from build123d import *

# Parameters (mm, degrees)
SKETCH1_W                                      = 50.8
SKETCH1_H                                      = 50.8
BOSS_EXTRUDE1_DEPTH                            = 6.35
CUT_EXTRUDE1_REACH                             = 38.478
SKETCH2_R                                      = 4.7625
SKETCH2_R_2                                    = 3.175
CUT_EXTRUDE2_REACH                             = 38.478
SKETCH5_R                                      = 1.4732
CSK_FOR_4_FLAT_HEAD_MACHINE_SCREW1_D           = 2.9464
CSK_FOR_4_FLAT_HEAD_MACHINE_SCREW1_CSINK_D     = 5.715
CSK_FOR_4_FLAT_HEAD_MACHINE_SCREW1_CSINK_ANGLE = 82
FILLET1_R                                      = 0.635


with BuildPart() as part:
    # Sketch1 → Boss-Extrude1 (new body)
    with BuildSketch(Plane(origin=(0, 0, 0), x_dir=(0, 1, 0), z_dir=(0, 0, 1))):
        Rectangle(SKETCH1_W, SKETCH1_H)
    extrude(amount=BOSS_EXTRUDE1_DEPTH)

    # Sketch2 → Cut-Extrude1 (cut, up to next)
    with BuildSketch(Plane.XY.offset(6.35), mode=Mode.PRIVATE) as cut_extrude1_sk1:
        with Locations((0, 8.73125)):
            Circle(SKETCH2_R)
    cut_extrude1_tool1 = extrude(cut_extrude1_sk1.sketch, amount=-CUT_EXTRUDE1_REACH, mode=Mode.PRIVATE) & part.part
    # Sketch2 → Cut-Extrude1 (cut, up to next)
    with BuildSketch(Plane.XY.offset(6.35), mode=Mode.PRIVATE) as cut_extrude1_sk2:
        with Locations((0, -8.73125)):
            Circle(SKETCH2_R_2)
    cut_extrude1_tool2 = extrude(cut_extrude1_sk2.sketch, amount=-CUT_EXTRUDE1_REACH, mode=Mode.PRIVATE) & part.part
    add(cut_extrude1_tool1.solids().sort_by_distance((0, 8.73125, 6.35))[0], mode=Mode.SUBTRACT)
    add(cut_extrude1_tool2.solids().sort_by_distance((0, -8.73125, 6.35))[0], mode=Mode.SUBTRACT)

    # Sketch5 → Cut-Extrude2 (cut, up to next)
    with BuildSketch(Plane.XY.offset(6.35), mode=Mode.PRIVATE) as cut_extrude2_sk1:
        with Locations((-20.32, 20.32)):
            Circle(SKETCH5_R)
    cut_extrude2_tool1 = extrude(cut_extrude2_sk1.sketch, amount=-CUT_EXTRUDE2_REACH, mode=Mode.PRIVATE) & part.part
    # Sketch5 → Cut-Extrude2 (cut, up to next)
    with BuildSketch(Plane.XY.offset(6.35), mode=Mode.PRIVATE) as cut_extrude2_sk2:
        with Locations((20.32, 20.32)):
            Circle(SKETCH5_R)
    cut_extrude2_tool2 = extrude(cut_extrude2_sk2.sketch, amount=-CUT_EXTRUDE2_REACH, mode=Mode.PRIVATE) & part.part
    # Sketch5 → Cut-Extrude2 (cut, up to next)
    with BuildSketch(Plane.XY.offset(6.35), mode=Mode.PRIVATE) as cut_extrude2_sk3:
        with Locations((-20.32, -20.32)):
            Circle(SKETCH5_R)
    cut_extrude2_tool3 = extrude(cut_extrude2_sk3.sketch, amount=-CUT_EXTRUDE2_REACH, mode=Mode.PRIVATE) & part.part
    # Sketch5 → Cut-Extrude2 (cut, up to next)
    with BuildSketch(Plane.XY.offset(6.35), mode=Mode.PRIVATE) as cut_extrude2_sk4:
        with Locations((20.32, -20.32)):
            Circle(SKETCH5_R)
    cut_extrude2_tool4 = extrude(cut_extrude2_sk4.sketch, amount=-CUT_EXTRUDE2_REACH, mode=Mode.PRIVATE) & part.part
    add(cut_extrude2_tool1.solids().sort_by_distance((-20.32, 20.32, 6.35))[0], mode=Mode.SUBTRACT)
    add(cut_extrude2_tool2.solids().sort_by_distance((20.32, 20.32, 6.35))[0], mode=Mode.SUBTRACT)
    add(cut_extrude2_tool3.solids().sort_by_distance((-20.32, -20.32, 6.35))[0], mode=Mode.SUBTRACT)
    add(cut_extrude2_tool4.solids().sort_by_distance((20.32, -20.32, 6.35))[0], mode=Mode.SUBTRACT)

    # CSK for #4 Flat Head Machine Screw1 (through all)
    with Locations(Plane.XY.offset(6.35)):
        with Locations((-20.32, 20.32), (20.32, 20.32), (20.32, -20.32), (-20.32, -20.32)):
            CounterSinkHole(CSK_FOR_4_FLAT_HEAD_MACHINE_SCREW1_D / 2, CSK_FOR_4_FLAT_HEAD_MACHINE_SCREW1_CSINK_D / 2, counter_sink_angle=CSK_FOR_4_FLAT_HEAD_MACHINE_SCREW1_CSINK_ANGLE)

    # Fillet1
    fillet1_edges = [part.edges().sort_by_distance(p)[0] for p in [
        (0, -25.4, 6.35),
        (25.4, 0, 6.35),
        (0, 25.4, 6.35),
        (25.4, 0, 0),
        (0, -25.4, 0),
        (-25.4, 0, 0),
        (0, 25.4, 0),
        (25.4, 25.4, 3.175),
        (25.4, -25.4, 3.175),
        (-25.4, -25.4, 3.175),
        (-25.4, 25.4, 3.175),
        (-25.4, 0, 6.35),
    ]]
    fillet(fillet1_edges, radius=FILLET1_R)


solid = part.part
Part model, mm, in its own coordinate system. Coordinates: 2 decimals unless noted, no trailing zeros. Order: outer loops, then holes, each group sorted by start corner. A loop starts at its lowest first (then second) coordinate and runs counter-clockwise, first axis right, second up.
(1) Probe L1, parallel to Y at x = 20.32, z = 2.1; L2, parallel to Y at x = -0.5, z = 1.75. List the from-to ranges inside material, lowest first.
Check sheet entries:
L1: y = -25.4 to -21.79, -18.85 to 18.85, 21.79 to 25.4
L2: y = -25.4 to -11.87, -5.6 to 4, 13.47 to 25.4
(2) Slice it at C-C, the plane y = 7.5. Write the cut outline in (x, z) (3 decimals), and give its area (3 significant figures).
Check sheet entries:
outline: (-25.4, 0.635) arc R0.635 ccw to (-24.765, 0) - (-4.601, 0) - (-4.601, 6.35) - (-24.765, 6.35) arc R0.635 ccw to (-25.4, 5.715) - close; (4.601, 0) - (24.765, 0) arc R0.635 ccw to (25.4, 0.635) - (25.4, 5.715) arc R0.635 ccw to (24.765, 6.35) - (4.601, 6.35) - close
area: 264 mm2
(3) Slice it at A-A, the plane x = -20.32. State how many separate pieces and enclosed holes the cut face has, and give its area (3 significant figures).
Check sheet entries:
separate pieces: 3
enclosed holes: 0
area: 280 mm2
(4) Pull direction X, two halves, no side cores. Call faces 1 (the face through (-25.4, 0, 3)), 2 (the face through (25.4, 0, 3)), 3 (the face through (19.151, -21.216, 2.412)), 4 (the face through (0, 25.4, 3)): pulls with the +X half, pulls with the -X half, needs draft (parallel to the pull), parting line crosses it, or undercut.
Check sheet entries:
face 1: pulls with the -X half
face 2: pulls with the +X half
face 3: undercut
face 4: needs draft
